```python
from build123d import *

# Parameters (mm, degrees)
SKETCH1_W = 5
SKETCH1_H = 43
SKETCH2_W = 1.75
SKETCH2_H = 1
FILLET1_R = 0.75
FILLET2_R = 0.25


with BuildPart() as part:
    # Sketch1 → Revolve1 (revolve)
    with BuildSketch(Plane.XY, mode=Mode.PRIVATE) as revolve1_sk:
        with Locations((-2.5, -21.5)):
            Rectangle(SKETCH1_W, SKETCH1_H)
    revolve(revolve1_sk.sketch.rotate(Axis((0, 0, 0), (0, -1, 0)), 270), axis=Axis((0, 0, 0), (0, -1, 0)))

    # Sketch2 → Revolve2 (revolve)
    with BuildSketch(Plane.XY, mode=Mode.PRIVATE) as revolve2_sk:
        with Locations((-0.875, 0.5)):
            Rectangle(SKETCH2_W, SKETCH2_H)
    revolve(revolve2_sk.sketch.rotate(Axis((0, 0, 0), (0, 1, 0)), 270), axis=Axis((0, 0, 0), (0, 1, 0)))

    # Fillet1
    fillet1_edges = [part.edges().sort_by_distance(p)[0] for p in [
        (0, 0, -5),
    ]]
    fillet(fillet1_edges, radius=FILLET1_R)

    # Fillet2
    fillet2_edges = [part.edges().sort_by_distance(p)[0] for p in [
        (0, 1, 1.75),
    ]]
    fillet(fillet2_edges, radius=FILLET2_R)


solid = part.part
```
For this review, take the finished solid that the model builds, in its own axes (mm). A direction names the side the tool comes from. Coordinates: 2 decimals unless noted, no trailing zeros. Write each loop counter-clockwise with the first axis right and the second up, starting at its lowest first coordinate (ties: lowest second). Pieces come first, ordered by that corner, then holes. Notation, with made-up numbers: (3.25, 74) - (38.25, 74) arc R14 cw to (38.25, 92) - close; hole circle Ø8 at (26.5, 77). An arc over 180 degrees is marked (long way). Answer in a Markdown table with one row per item. Add a question column.
Q1. We need section A-A, the plane z = 0. State the section outline as (x, y) points.
Q2. We need section C-C, the plane y = -10.5. State the section outline as (x, z) points, and give its area (3 significant figures).
Q3. For probe 1 along Y at (x, z) = (-0.25, -2.75); probe 2 along X at (y, z) = (-4.5, -0.25), list the stretches that pass through material, from the lowest coordinate up.
Q4. For P1, Ø1, axis at y = -27.5, z = 1.5, coming from the +X side; P2, Ø1, axis at y = -33.5, z = -3, coming from the +X side, all flat-tipped, find the tip position at first contact; note any pin that passes through.
Q5. Tool access review of faces 1 (the flat face through (0, 0, 2)), 2 (the flat face through (0, -43, 0)): name each direction out of +Z, -Z, +X, -X, +Y, -Y from which nothing blocks a thin tool from reaching the whole face with its end or side.
Q6. We need section B-B, the plane x = 0. State the section outline as (y, z) points.
Answer list:
| question | item | result |
|---|---|---|
| 1 | outline | (-5, -43) - (5, -43) - (5, -0.75) arc R0.75 ccw to (4.25, 0) - (1.75, 0) - (1.75, 0.75) arc R0.25 ccw to (1.5, 1) - (-1.5, 1) arc R0.25 ccw to (-1.75, 0.75) - (-1.75, 0) - (-4.25, 0) arc R0.75 ccw to (-5, -0.75) - close |
| 2 | outline | circle Ø10 at (0, 0) |
| 2 | area | 78.5 mm2 |
| 3 | probe 1 | y = -43 to 0 |
| 3 | probe 2 | x = -4.99 to 4.99 |
| 4 | P1 | stops at x = 4.9 |
| 4 | P2 | stops at x = 4.33 |
| 5 | face 1 | +Y |
| 5 | face 2 | +Z, -Z, +X, -X, -Y |
| 6 | outline | (-43, -5) - (-0.75, -5) arc R0.75 ccw to (0, -4.25) - (0, -1.75) - (0.75, -1.75) arc R0.25 ccw to (1, -1.5) - (1, 1.5) arc R0.25 ccw to (0.75, 1.75) - (0, 1.75) - (0, 4.25) arc R0.75 ccw to (-0.75, 5) - (-43, 5) - close |
